Verification items for the finished model (mm, model axes). Face numbers are marked on the shaded views. Give positions to 0.01 mm unless a question says otherwise; leave off trailing zeros. Loops run counter-clockwise (first coordinate to the right, second up) from the corner with the lowest first, then second, coordinate; pieces in that order, holes last. Notation, with made-up numbers: M 51,52.25 L 74,52.25 A26 ccw 74,79.25 Z; hole C 69.5,-16.75 d10. An arc over 180 degrees is marked long. Answer in a Markdown table with one row per item.
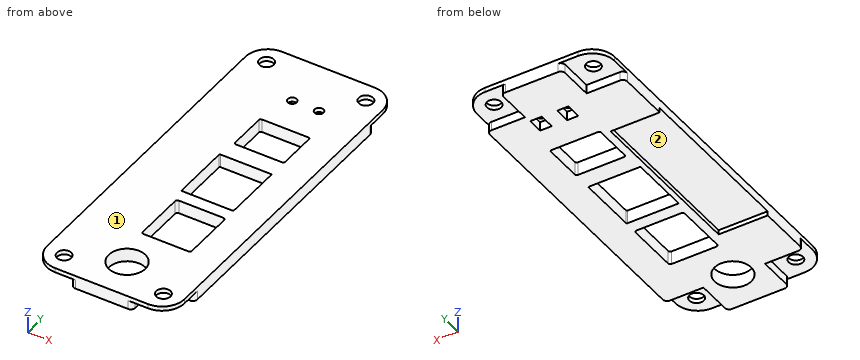
```python
from build123d import *

# Parameters (mm, degrees)
SKETCH_1_R          = 1
EXTRUDE_1_DEPTH     = 3
SKETCH_2_W          = 11
SKETCH_2_H          = 38
CUT_EXTRUDE_1_DEPTH = 1
CUT_EXTRUDE_START   = -2
CUT_EXTRUDE_2_DEPTH = 2
SKETCH_4_R          = 1.6
CUT_EXTRUDE_3_DEPTH = 62.990079852
SKETCH_6_W          = 2.6
SKETCH_6_H          = 3.5
SKETCH_6_W_2        = 2.5
CUT_EXTRUDE_4_DEPTH = 2
SKETCH_7_R          = 4.1
CUT_EXTRUDE_5_DEPTH = 63.030395775
FILLET_1_R          = 1


with BuildPart() as part:
    # 草图1 → 凸台-拉伸1 (new body)
    with BuildSketch(Plane.XY):
        with BuildLine():
            Line((47.4, -34.9), (47.4, 34.9))
            ThreePointArc((47.4, 34.9), (45.935533906, 38.435533906), (42.4, 39.9))
            Line((42.4, 39.9), (21.6, 39.9))
            ThreePointArc((21.6, 39.9), (18.064466094, 38.435533906), (16.6, 34.9))
            Line((16.6, 34.9), (16.6, -34.9))
            ThreePointArc((16.6, -34.9), (18.064466094, -38.435533906), (21.6, -39.9))
            Line((21.6, -39.9), (42.4, -39.9))
            ThreePointArc((42.4, -39.9), (45.935533906, -38.435533906), (47.4, -34.9))
        make_face()
        with Locations((37.413843028, 28.102429875)):
            Circle(SKETCH_1_R, mode=Mode.SUBTRACT)
        with Locations((31.413843028, 28.102429875)):
            Circle(SKETCH_1_R, mode=Mode.SUBTRACT)
        with BuildLine():
            Line((40.513850359, -21.477641558), (40.513850359, -10.127641653))
            ThreePointArc((40.513850359, -10.127641653), (40.367403749, -9.774088262), (40.013850359, -9.627641653))
            Line((40.013850359, -9.627641653), (30.013850359, -9.627641653))
            ThreePointArc((30.013850359, -9.627641653), (29.660296968, -9.774088262), (29.513850359, -10.127641653))
            Line((29.513850359, -10.127641653), (29.513850359, -21.477641558))
            ThreePointArc((29.513850359, -21.477641558), (29.660296968, -21.831194949), (30.013850359, -21.977641558))
            Line((30.013850359, -21.977641558), (40.013850359, -21.977641558))
            ThreePointArc((40.013850359, -21.977641558), (40.367403749, -21.831194949), (40.513850359, -21.477641558))
        make_face(mode=Mode.SUBTRACT)
        with BuildLine():
            Line((40.464996896, 6.495389649), (40.464996896, -6.604609867))
            ThreePointArc((40.464996896, -6.604609867), (40.406418252, -6.746031223), (40.264996896, -6.804609867))
            Line((40.264996896, -6.804609867), (28.963873947, -6.804609867))
            ThreePointArc((28.963873947, -6.804609867), (28.822452591, -6.746031223), (28.763873947, -6.604609867))
            Line((28.763873947, -6.604609867), (28.763873947, 6.495389649))
            ThreePointArc((28.763873947, 6.495389649), (28.822452591, 6.636811005), (28.963873947, 6.695389649))
            Line((28.963873947, 6.695389649), (40.264996896, 6.695389649))
            ThreePointArc((40.264996896, 6.695389649), (40.406418252, 6.636811005), (40.464996896, 6.495389649))
        make_face(mode=Mode.SUBTRACT)
        with BuildLine():
            Line((40.513843009, 11.302412116), (40.513843009, 19.702429875))
            ThreePointArc((40.513843009, 19.702429875), (40.396685721, 19.985272588), (40.113843009, 20.102429875))
            Line((40.113843009, 20.102429875), (29.713821303, 20.102429875))
            ThreePointArc((29.713821303, 20.102429875), (29.43097859, 19.985272588), (29.313821303, 19.702429875))
            Line((29.313821303, 19.702429875), (29.313821303, 11.302412116))
            ThreePointArc((29.313821303, 11.302412116), (29.43097859, 11.019569403), (29.713821303, 10.902412116))
            Line((29.713821303, 10.902412116), (40.113843009, 10.902412116))
            ThreePointArc((40.113843009, 10.902412116), (40.396685721, 11.019569403), (40.513843009, 11.302412116))
        make_face(mode=Mode.SUBTRACT)
    extrude(amount=-EXTRUDE_1_DEPTH)

    # 草图2 → 切除-拉伸1 (cut)
    with BuildSketch(Plane(origin=(0, 0, -3), x_dir=(-1, 0, 0), z_dir=(0, 0, -1))):
        with Locations((-22.1, 0)):
            Rectangle(SKETCH_2_W, SKETCH_2_H)
    extrude(amount=-CUT_EXTRUDE_1_DEPTH, mode=Mode.SUBTRACT)

    # 草图3 → 切除-拉伸2 (cut)
    with BuildSketch(Plane(origin=(0, 0, -3), x_dir=(-1, 0, 0), z_dir=(0, 0, -1)).offset(CUT_EXTRUDE_START)):
        with BuildLine():
            Line((-47.4, -31.4), (-38.9, -31.4))
            Line((-38.9, -31.4), (-38.9, -39.9))
            Line((-38.9, -39.9), (-42.4, -39.9))
            ThreePointArc((-42.4, -39.9), (-45.935533906, -38.435533906), (-47.4, -34.9))
            Line((-47.4, -34.9), (-47.4, -31.4))
        make_face()
        with BuildLine():
            Line((-47.4, 34.9), (-47.4, 31.4))
            Line((-47.4, 31.4), (-38.9, 31.4))
            Line((-38.9, 31.4), (-38.9, 39.9))
            Line((-38.9, 39.9), (-42.4, 39.9))
            ThreePointArc((-42.4, 39.9), (-45.935533906, 38.435533906), (-47.4, 34.9))
        make_face()
        with BuildLine():
            Line((-16.6, 31.4), (-25.1, 31.4))
            Line((-25.1, 31.4), (-25.1, 39.9))
            Line((-25.1, 39.9), (-21.6, 39.9))
            ThreePointArc((-21.6, 39.9), (-18.064466094, 38.435533906), (-16.6, 34.9))
            Line((-16.6, 34.9), (-16.6, 31.4))
        make_face()
        with BuildLine():
            Line((-16.6, -34.9), (-16.6, -31.4))
            Line((-16.6, -31.4), (-25.1, -31.4))
            Line((-25.1, -31.4), (-25.1, -39.9))
            Line((-25.1, -39.9), (-21.6, -39.9))
            ThreePointArc((-21.6, -39.9), (-18.064466094, -38.435533906), (-16.6, -34.9))
        make_face()
    extrude(amount=CUT_EXTRUDE_2_DEPTH, mode=Mode.SUBTRACT)

    # 草图4 → 切除-拉伸3 (cut, through all)
    with BuildSketch(Plane(origin=(0, 0, -1), x_dir=(-1, 0, 0), z_dir=(0, 0, -1))):
        with Locations((-20.872307757, 35.627692243)):
            Circle(SKETCH_4_R)
        with Locations(Location((-20.872307757, -35.627692243, 0), (0, 0, 180))):
            Circle(SKETCH_4_R)
        with Locations((-43.127692243, -35.627692243)):
            Circle(SKETCH_4_R)
        with Locations(Location((-43.127692243, 35.627692243, 0), (0, 0, 180))):
            Circle(SKETCH_4_R)
    extrude(amount=-CUT_EXTRUDE_3_DEPTH, mode=Mode.SUBTRACT)

    # 草图6 → 切除-拉伸4 (cut)
    with BuildSketch(Plane(origin=(0, 0, -3), x_dir=(-1, 0, 0), z_dir=(0, 0, -1))):
        with Locations((-37.413843028, 28.102429875)):
            Rectangle(SKETCH_6_W, SKETCH_6_H)
        with Locations((-31.413843028, 28.102429875)):
            Rectangle(SKETCH_6_W_2, SKETCH_6_H)
    extrude(amount=-CUT_EXTRUDE_4_DEPTH, mode=Mode.SUBTRACT)

    # 草图7 → 切除-拉伸5 (cut, through all)
    with BuildSketch(Plane.XY):
        with Locations((32, -30.938820779)):
            Circle(SKETCH_7_R)
    extrude(amount=-CUT_EXTRUDE_5_DEPTH, mode=Mode.SUBTRACT)

    # 圆角1
    fillet_1_edges = [part.edges().sort_by_distance(p)[0] for p in [
        (25.1, -39.9, -2),
        (16.6, -31.4, -2),
        (16.6, 31.4, -2),
        (25.1, 39.9, -2),
        (38.9, 39.9, -2),
        (47.4, 31.4, -2),
        (47.4, -31.4, -2),
        (38.9, -39.9, -2),
    ]]
    fillet(fillet_1_edges, radius=FILLET_1_R)


solid = part.part
```
Item 1: Sectioned sample at C-C (z = -2.55). State how many separate pieces and enclosed holes the cut face has, and give its area (3 significant figures).
Reported:
| item | result |
|---|---|
| separate pieces | 1 |
| enclosed holes | 6 |
| area | 1,280 mm^2 |
Item 2: Sectioned sample at A-A (y = 5). Record the cut outline in (x, z) (3 decimals), and give its area (3 significant figures).
Reported:
| item | result |
|---|---|
| outline | M 16.6,-2 L 27.6,-2 L 27.6,-3 L 28.764,-3 L 28.764,0 L 16.6,0 Z; M 40.465,-3 L 47.4,-3 L 47.4,0 L 40.465,0 Z |
| area | 46.3 mm^2 |
Item 3: Go/stop test with flat-tipped pins: pin 1 (3 mm diameter, centred on x = 21, y = 34.5, fed in from -Z); pin 2 (1.6 mm diameter, centred on y = 33.5, z = -2.5, fed in from -X); pin 3 (0.5 mm diameter, centred on x = 20.5, z = -2.5, fed in from -Y); pin 4 (3.5 mm diameter, centred on x = 43.13, y = -35.63, fed in from +Z). Record where each tip stops, or that it passes through.
Reported:
| item | result |
|---|---|
| pin 1 | stops at z = -1 |
| pin 2 | stops at x = 25.1 |
| pin 3 | stops at y = -31.4 |
| pin 4 | stops at z = 0 |
Item 4: Scan lines: L1, parallel to Y at x = 39, z = -0.4; L2, parallel to Y at x = 40, z = -1.5; L3, parallel to X at y = 3.5, z = -0.7 (3 decimals). Record each from-to range of solid material in increasing order. Write a range as [from, to].
Reported:
| item | result |
|---|---|
| L1 | y = [-39.9, -21.98], [-9.63, -6.8], [6.7, 10.9], [20.1, 39.9] |
| L2 | y = [-31.4, -21.98], [-9.63, -6.8], [6.7, 10.9], [20.1, 31.4] |
| L3 | x = [16.6, 28.764], [40.465, 47.4] |
Item 5: Sectioned sample at D-D (y = -29). Record the cut outline in (x, z), and give its area (3 significant figures).
Reported:
| item | result |
|---|---|
| outline | M 16.6,-3 L 28.39,-3 L 28.39,0 L 16.6,0 Z; M 35.61,-3 L 47.4,-3 L 47.4,0 L 35.61,0 Z |
| area | 70.7 mm^2 |
Item 6: Release check for a two-part mould opening along Y. For the marked faces 1 and 2 record: released by +Y, released by -Y, zero draft, split by the parting line, or undercut.
Reported:
| item | result |
|---|---|
| face 1 | zero draft |
| face 2 | undercut |
Item 7: Sectioned sample at B-B (x = 34). Record the cut outline in (y, z).
Reported:
| item | result |
|---|---|
| outline | M -39.9,-3 L -34.52,-3 L -34.52,0 L -39.9,0 Z; M -27.36,-3 L -21.98,-3 L -21.98,0 L -27.36,0 Z; M -9.63,-3 L -6.8,-3 L -6.8,0 L -9.63,0 Z; M 6.7,-3 L 10.9,-3 L 10.9,0 L 6.7,0 Z; M 20.1,-3 L 39.9,-3 L 39.9,0 L 20.1,0 Z |
